from build123d import *

# Parameters (mm, degrees)
SKETCH1_W           = 71
SKETCH1_H           = 39
BOSS_EXTRUDE1_DEPTH = 31
SHELL1_T            = -2
CUT_EXTRUDE1_DEPTH  = 52.004901725
SKETCH4_W           = 20
SKETCH4_H           = 5
CUT_EXTRUDE2_DEPTH  = 27
SKETCH5_W           = 5
SKETCH5_H           = 2
CUT_EXTRUDE3_DEPTH  = 52.004901725
FILLET2_R           = 3


with BuildPart() as part:
    # Sketch1 → Boss-Extrude1 (new body)
    with BuildSketch(Plane(origin=(0, 0, 0), x_dir=(1, 0, 0), z_dir=(0, 1, 0))):
        Rectangle(SKETCH1_W, SKETCH1_H)
    extrude(amount=BOSS_EXTRUDE1_DEPTH)

    # Shell1
    shell1_openings = [part.faces().sort_by_distance(p)[0] for p in [
        (0, 0, 0),
    ]]
    offset(amount=SHELL1_T, openings=shell1_openings, kind=Kind.INTERSECTION)

    # Sketch2 → Cut-Extrude1 (cut, through all)
    with BuildSketch(Plane(origin=(0, 31, 0), x_dir=(1, 0, 0), z_dir=(0, 1, 0))):
        Polygon((-29.160254038, 19.5), (5, 19.5), (5, 14.5), (-20.5, 14.5), align=None)
        Polygon((-20.5, -14.5), (5, -14.5), (5, -19.5), (-29.160254038, -19.5), align=None)
    extrude(amount=-CUT_EXTRUDE1_DEPTH, mode=Mode.SUBTRACT)

    # Sketch4 → Cut-Extrude2 (cut)
    with BuildSketch(Plane(origin=(0, 31, -31), x_dir=(1, 0, 0), z_dir=(0, -1, 0))):
        with Locations((25.5, 48)):
            Rectangle(SKETCH4_W, SKETCH4_H)
        with Locations((25.5, 14)):
            Rectangle(SKETCH4_W, SKETCH4_H)
    extrude(amount=CUT_EXTRUDE2_DEPTH, mode=Mode.SUBTRACT)

    # Sketch5 → Cut-Extrude3 (cut, through all)
    with BuildSketch(Plane(origin=(0, 31, 0), x_dir=(1, 0, 0), z_dir=(0, 1, 0))):
        with Locations((-28, 15.5)):
            Rectangle(SKETCH5_W, SKETCH5_H)
        with Locations((11, 16)):
            Rectangle(SKETCH5_W, SKETCH5_H)
        with Locations((11, -16)):
            Rectangle(SKETCH5_W, SKETCH5_H)
        with Locations((-28, -15.5)):
            Rectangle(SKETCH5_W, SKETCH5_H)
    extrude(amount=-CUT_EXTRUDE3_DEPTH, mode=Mode.SUBTRACT)

    # Fillet2
    fillet2_edges = [part.edges().sort_by_distance(p)[0] for p in [
        (-35.5, 15.5, 19.5),
        (-35.5, 15.5, -19.5),
    ]]
    fillet(fillet2_edges, radius=FILLET2_R)


solid = part.part
Geometry: final body of the model. Coordinates: model frame, mm. A direction names the side the tool comes from. Round coordinates to 2 decimals unless told otherwise and drop trailing zeros. Order: outer loops, then holes, each group sorted by start corner. A loop starts at its lowest first (then second) coordinate and runs counter-clockwise, first axis right, second up.
Q1. Section C-C, the plane z = -7.5. Output: boundary loops of the cut face in (x, y), and give its area (3 significant figures).
Result sheet:
outline: (-35.5, 0) - (-33.5, 0) - (-33.5, 29) - (33.5, 29) - (33.5, 0) - (35.5, 0) - (35.5, 31) - (-35.5, 31) - close
area: 258 mm2
Q2. Section A-A, the plane y = 24.5. Output: boundary loops of the cut face in (x, z).
Result sheet:
outline: (-35.5, -16.5) arc R3 ccw to (-32.5, -19.5) - (-29.16, -19.5) - (-25.7, -17.5) - (-33.5, -17.5) - (-33.5, 17.5) - (-25.7, 17.5) - (-29.16, 19.5) - (-32.5, 19.5) arc R3 ccw to (-35.5, 16.5) - close; (5, -19.5) - (15.5, -19.5) - (15.5, -17.5) - (5, -17.5) - close; (5, 17.5) - (15.5, 17.5) - (15.5, 19.5) - (5, 19.5) - close; (33.5, -14.5) - (35.5, -14.5) - (35.5, 14.5) - (33.5, 14.5) - close
Q3. Section D-D, the plane x = 1. Output: boundary loops of the cut face in (y, z).
Result sheet:
outline: (29, -14.5) - (31, -14.5) - (31, 14.5) - (29, 14.5) - close
Q4. Mould query, pull axis Z, two halves, no side actions, for faces 6 (the face through (-31, 15, 19.5)), 7 (the face through (-30, 14, -17.5)), 8 (the face through (11, 30, -15)), 9 (the face through (-34, 0, 1)). Classes: released by +Z, released by -Z, zero draft, split by the parting line, or undercut.
Result sheet:
face 6: released by +Z
face 7: undercut
face 8: undercut
face 9: zero draft
Q5. Material intervals for probe 1 along Z at (x, y) = (7, 10); probe 2 along X at (y, z) = (9.5, -6.5); probe 3 along Y at (x, z) = (-5.5, -3.5), sorted ascending.
Result sheet:
probe 1: z = -19.5 to -17.5, 17.5 to 19.5
probe 2: x = -35.5 to -33.5, 33.5 to 35.5
probe 3: y = 29 to 31
Q6. Section B-B, the plane x = 25. Output: boundary loops of the cut face in (y, z), and give its area (3 significant figures).
Result sheet:
outline: (0, -19.5) - (4, -19.5) - (4, -17.5) - (0, -17.5) - close; (0, 17.5) - (4, 17.5) - (4, 19.5) - (0, 19.5) - close; (29, -14.5) - (31, -14.5) - (31, 14.5) - (29, 14.5) - close
area: 74.0 mm2
Q7. Access query for faces 1 (the face through (15.5, 18, -18)), 2 (the face through (8.5, 30, 16)), 3 (the face through (-33.5, 14, 0)), 4 (the face through (5, 16, 18)), 5 (the face through (5, 16, -18)). Directions: +Z, -Z, +X, -X, +Y, -Y. A direction counts if a zero-diameter tool reaches every point of the face in a straight line with its end or side. Return the directions, or none.
Result sheet:
face 1: -Z, +X, +Y
face 2: +Y, -Y
face 3: -Y
face 4: +Z, +Y, -Y
face 5: -Z, +Y, -Y
Q8. Pin query (flat end, axial travel): pin 1 (10 mm diameter, centred on x = 26.5, y = 14, fed in from +Z); pin 2 (8.5 mm diameter, centred on x = -28, y = 13, fed in from +Z); pin 3 (2 mm diameter, centred on y = 30.5, z = -16, fed in from +X); pin 4 (1 mm diameter, centred on x = -5.5, y = 30, fed in from -Z). Return the tip coordinate at first contact, or that it passes through.
Result sheet:
pin 1: passes through
pin 2: stops at z = 19.5
pin 3: stops at x = 15.5
pin 4: stops at z = -14.5
